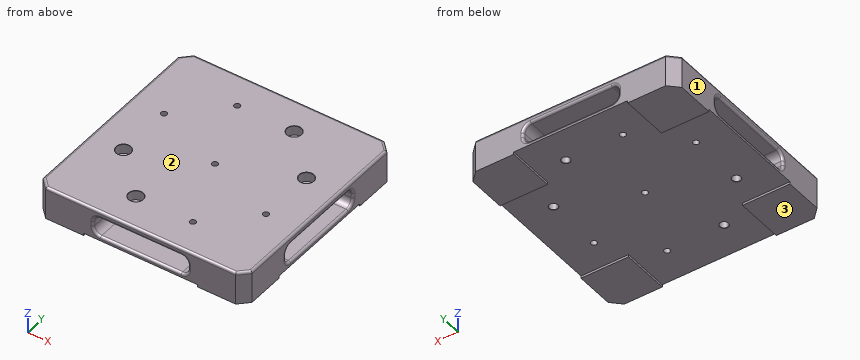
from build123d import *

# Parameters (mm, degrees)
BOSS_EXTRUDE1_DEPTH                           = 40.64
F_3_8_16_TAPPED_HOLE1_D                       = 7.9375
CBORE_FOR_3_8_SOCKET_HEAD_CAP_SCREW1_AT_COUNT = 2
CBORE_FOR_3_8_SOCKET_HEAD_CAP_SCREW1_AT_PITCH = 188.585378542
CBORE_FOR_3_8_SOCKET_HEAD_CAP_SCREW1_2_COUNT  = 2
CBORE_FOR_3_8_SOCKET_HEAD_CAP_SCREW1_2_PITCH  = 80.82230509
CBORE_FOR_3_8_SOCKET_HEAD_CAP_SCREW1_3_COUNT  = 2
CBORE_FOR_3_8_SOCKET_HEAD_CAP_SCREW1_3_PITCH  = 205.174779152
FILLET1_R                                     = 3.175
CUT_EXTRUDE2_DEPTH                            = 28.448
FILLET2_R                                     = 3.175
CIRPATTERN1_COUNT                             = 4
FILLET2_OF_CIRPATTERN1_R                      = 3.175
BOSS_EXTRUDE2_DEPTH                           = 3.175


with BuildPart() as part:
    # Sketch1 → Boss-Extrude1 (new body)
    with BuildSketch(Plane.XY):
        Polygon((-127, 139.7), (127, 139.7), (139.7, 127), (139.7, -127), (127, -139.7), (-127, -139.7), (-139.7, -127), (-139.7, 127), align=None)
    extrude(amount=BOSS_EXTRUDE1_DEPTH)

    # 3_8-16 Tapped Hole1 (through all)
    with Locations(Plane.XY.offset(40.64)):
        with Locations((-95.25, 38.1), (-38.1, 95.25), (38.1, -95.25), (95.25, -38.1), (0, 0)):
            Hole(F_3_8_16_TAPPED_HOLE1_D / 2)

    # Sketch7 → CBORE for 3_8 Socket Head Cap Screw1 (revolve, cut)
    with BuildSketch(Plane(origin=(-95.25, -38.1, 40.64), x_dir=(0, -1, 0), z_dir=(1, 0, 0))):
        Polygon((0, 0), (0, 40.64), (5.8674, 40.64), (5.4483, 40.2209), (5.4483, 12.7), (9.525, 12.7), (9.525, 0.381), (9.906, 0), align=None)
    cbore_for_3_8_socket_head_cap_screw1 = revolve(axis=Axis((-95.25, -38.1, 46.99), (0, 0, -1)), mode=Mode.SUBTRACT)

    # CBORE for 3_8 Socket Head Cap Screw1 at: CBORE for 3_8 Socket Head Cap Screw1 ×2
    with Locations(*[Vector(0.707106781, 0.707106781, 0) * (i * CBORE_FOR_3_8_SOCKET_HEAD_CAP_SCREW1_AT_PITCH) for i in range(1, CBORE_FOR_3_8_SOCKET_HEAD_CAP_SCREW1_AT_COUNT)]):
        add(cbore_for_3_8_socket_head_cap_screw1, mode=Mode.SUBTRACT)

    # CBORE for 3_8 Socket Head Cap Screw1 2: CBORE for 3_8 Socket Head Cap Screw1 ×2
    with Locations(*[Vector(0.707106781, -0.707106781, 0) * (i * CBORE_FOR_3_8_SOCKET_HEAD_CAP_SCREW1_2_PITCH) for i in range(1, CBORE_FOR_3_8_SOCKET_HEAD_CAP_SCREW1_2_COUNT)]):
        add(cbore_for_3_8_socket_head_cap_screw1, mode=Mode.SUBTRACT)

    # CBORE for 3_8 Socket Head Cap Screw1 3: CBORE for 3_8 Socket Head Cap Screw1 ×2
    with Locations(*[Vector(0.928476691, 0.371390676, 0) * (i * CBORE_FOR_3_8_SOCKET_HEAD_CAP_SCREW1_3_PITCH) for i in range(1, CBORE_FOR_3_8_SOCKET_HEAD_CAP_SCREW1_3_COUNT)]):
        add(cbore_for_3_8_socket_head_cap_screw1, mode=Mode.SUBTRACT)

    # Fillet1
    fillet1_edges = [part.edges().sort_by_distance(p)[0] for p in [
        (-133.35, -133.35, 40.64),
        (0, -139.7, 40.64),
        (133.35, -133.35, 40.64),
        (139.7, 0, 40.64),
        (133.35, 133.35, 40.64),
        (0, 139.7, 40.64),
        (-133.35, 133.35, 40.64),
        (-139.7, 0, 40.64),
    ]]
    fillet(fillet1_edges, radius=FILLET1_R)

    # Sketch9 → Cut-Extrude2 (cut)
    with BuildSketch(Plane.XZ.offset(139.7)):
        with BuildLine():
            Line((-53.975, 31.115), (53.975, 31.115))
            ThreePointArc((53.975, 31.115), (60.710192091, 28.325192091), (63.5, 21.59))
            Line((63.5, 21.59), (63.5, 15.24))
            ThreePointArc((63.5, 15.24), (60.710192091, 8.504807909), (53.975, 5.715))
            Line((53.975, 5.715), (-53.975, 5.715))
            ThreePointArc((-53.975, 5.715), (-60.710192091, 8.504807909), (-63.5, 15.24))
            Line((-63.5, 15.24), (-63.5, 21.59))
            ThreePointArc((-63.5, 21.59), (-60.710192091, 28.325192091), (-53.975, 31.115))
        make_face()
    cut_extrude2 = extrude(amount=-CUT_EXTRUDE2_DEPTH, mode=Mode.SUBTRACT)

    # Fillet2
    fillet2_edges = [part.edges().sort_by_distance(p)[0] for p in [
        (60.710192091, -139.7, 28.325192091),
        (0, -139.7, 31.115),
        (-60.710192091, -139.7, 28.325192091),
        (-63.5, -139.7, 18.415),
        (-60.710192091, -139.7, 8.504807909),
        (0, -139.7, 5.715),
        (60.710192091, -139.7, 8.504807909),
        (63.5, -139.7, 18.415),
    ]]
    fillet(fillet2_edges, radius=FILLET2_R)

    # CirPattern1: Cut-Extrude2 ×4 about axis
    cirpattern1_axis = Axis((0, 0, 0), (0, 0, 1))
    for i in range(1, CIRPATTERN1_COUNT):
        add(cut_extrude2.rotate(cirpattern1_axis, i * 360 / CIRPATTERN1_COUNT), mode=Mode.SUBTRACT)

    # Fillet2 of CirPattern1
    fillet2_of_cirpattern1_edges = [part.edges().sort_by_distance(p)[0] for p in [
        (139.7, 60.710192091, 28.325192091),
        (139.7, 0, 31.115),
        (139.7, -60.710192091, 28.325192091),
        (139.7, -63.5, 18.415),
        (139.7, -60.710192091, 8.504807909),
        (139.7, 0, 5.715),
        (139.7, 60.710192091, 8.504807909),
        (139.7, 63.5, 18.415),
        (-60.710192091, 139.7, 28.325192091),
        (0, 139.7, 31.115),
        (60.710192091, 139.7, 28.325192091),
        (63.5, 139.7, 18.415),
        (60.710192091, 139.7, 8.504807909),
        (0, 139.7, 5.715),
        (-60.710192091, 139.7, 8.504807909),
        (-63.5, 139.7, 18.415),
        (-139.7, -60.710192091, 28.325192091),
        (-139.7, 0, 31.115),
        (-139.7, 60.710192091, 28.325192091),
        (-139.7, 63.5, 18.415),
        (-139.7, 60.710192091, 8.504807909),
        (-139.7, 0, 5.715),
        (-139.7, -60.710192091, 8.504807909),
        (-139.7, -63.5, 18.415),
    ]]
    fillet(fillet2_of_cirpattern1_edges, radius=FILLET2_OF_CIRPATTERN1_R)

    # Sketch2 → Boss-Extrude2 (add)
    with BuildSketch(Plane(origin=(0, 0, 0), x_dir=(-1, 0, 0), z_dir=(0, 0, -1))):
        Polygon((127, -139.7), (76.2, -139.7), (76.2, -76.2), (139.7, -76.2), (139.7, -127), align=None)
        Polygon((-76.2, -139.7), (-127, -139.7), (-139.7, -127), (-139.7, -76.2), (-76.2, -76.2), align=None)
        Polygon((139.7, 76.2), (76.2, 76.2), (76.2, 139.7), (127, 139.7), (139.7, 127), align=None)
        Polygon((-127, 139.7), (-76.2, 139.7), (-76.2, 76.2), (-139.7, 76.2), (-139.7, 127), align=None)
    extrude(amount=BOSS_EXTRUDE2_DEPTH)


solid = part.part
Here's how the part is built. I have some questions about the finished solid (model axes, mm). Face numbers are marked on the shaded views. Round coordinates to 2 decimals unless told otherwise and drop trailing zeros. Write each loop counter-clockwise with the first axis right and the second up, starting at its lowest first coordinate (ties: lowest second). Pieces come first, ordered by that corner, then holes.
1. I need wall thicknesses on L1, parallel to Y at x = -95.25, z = 13.25; L2, parallel to X at y = 38, z = 15; L3, parallel to X at y = -38, z = 12.5. Which ranges of each line are inside material? Lowest first, please.
2. If we mould it in two halves opening along Z, with no side actions, what happens to the marked faces 1, 2 and 3? For each: released by +Z, released by -Z, zero draft, split by the parting line, or undercut.
3. Suppose I cut it at B-B (y = -95.25). List the corners of the cut face in (x, z) for me (3 decimals).
4. Suppose I cut it at D-D (y = 0). List the corners of the cut face in (x, z) for me (3 decimals).
5. Suppose I cut it at A-A (x = 118). List the corners of the cut face in (y, z) for me (3 decimals), and give its area (3 significant figures).
6. Will these pins go through, and if not, where does the flat tip stop? pin 1 Ø8 at (y, z) = (-48.5, 10.5) entering from -X; pin 2 Ø12 at (y, z) = (54.5, 27.5) entering from +X; pin 3 Ø17 at (x, y) = (38.1, 95.25) entering from +Z.
Answer sheet:
1. L1: y = -139.7 to -43.55, -32.65 to 34.13, 42.07 to 139.7
1. L2: x = -111.25 to -99.22, -91.28 to 89.8, 100.7 to 111.25
1. L3: x = -111.25 to -100.7, -89.8 to 91.28, 99.22 to 111.25
2. face 1: zero draft
2. face 2: released by +Z
2. face 3: released by -Z
3. outline: (-139.7, -3.175) - (-76.2, -3.175) - (-76.2, 0) - (-43.967, 0) - (-43.548, 0.419) - (-43.548, 27.94) - (-47.625, 27.94) - (-47.625, 40.259) - (-48.006, 40.64) - (-136.525, 40.64) arc R3.175 ccw to (-139.7, 37.465) - close; (-32.652, 0.419) - (-32.233, 0) - (34.131, 0) - (34.131, 40.64) - (-28.194, 40.64) - (-28.575, 40.259) - (-28.575, 27.94) - (-32.652, 27.94) - close; (42.069, 0) - (76.2, 0) - (76.2, -3.175) - (139.7, -3.175) - (139.7, 37.465) arc R3.175 ccw to (136.525, 40.64) - (42.069, 40.64) - close
4. outline: (-139.7, 0) - (-3.969, 0) - (-3.969, 40.64) - (-136.525, 40.64) arc R3.175 ccw to (-139.7, 37.465) - (-139.7, 34.29) arc R3.175 ccw to (-136.525, 31.115) - (-111.252, 31.115) - (-111.252, 5.715) - (-136.525, 5.715) arc R3.175 ccw to (-139.7, 2.54) - close; (3.969, 0) - (139.7, 0) - (139.7, 2.54) arc R3.175 ccw to (136.525, 5.715) - (111.252, 5.715) - (111.252, 31.115) - (136.525, 31.115) arc R3.175 ccw to (139.7, 34.29) - (139.7, 37.465) arc R3.175 ccw to (136.525, 40.64) - (3.969, 40.64) - close
5. outline: (-139.7, -3.175) - (-76.2, -3.175) - (-76.2, 0) - (76.2, 0) - (76.2, -3.175) - (139.7, -3.175) - (139.7, 37.465) arc R3.175 ccw to (136.525, 40.64) - (-136.525, 40.64) arc R3.175 ccw to (-139.7, 37.465) - close; hole (-63.5, 15.24) arc R9.525 ccw to (-53.975, 5.715) - (53.975, 5.715) arc R9.525 ccw to (63.5, 15.24) - (63.5, 21.59) arc R9.525 ccw to (53.975, 31.115) - (-53.975, 31.115) arc R9.525 ccw to (-63.5, 21.59) - close
5. area: 8,610 mm2
6. pin 1: stops at x = -111.25
6. pin 2: stops at x = 139.61
6. pin 3: stops at z = 27.94
